Verification items for the finished model (mm, model axes). A direction names the side the tool comes from. Round coordinates to 2 decimals unless told otherwise and drop trailing zeros. Write each loop counter-clockwise with the first axis right and the second up, starting at its lowest first coordinate (ties: lowest second). Pieces come first, ordered by that corner, then holes. Notation, with made-up numbers: M -29,43 L 1,43 A10 cw 1,51 Z; hole C 89,86 d6. An arc over 180 degrees is marked long. Answer in a Markdown table with one row per item. Add a question column.
1. Sectioned sample at B-B on y = -3. Record the cut outline in (x, z).
2. Material ranges on probe 1 along X at (y, z) = (-22.5, 15); probe 2 along Y at (x, z) = (74, 22.5); probe 3 along X at (y, z) = (-13.5, 2), recorded low to high.
3. Sectioned sample at A-A on x = 75.5. Record the cut outline in (y, z).
4. Go/stop test with flat-tipped pins: pin 1 Ø10 at (x, y) = (48, -31.5) entering from +Z; pin 2 Ø10 at (x, y) = (40, -26) entering from +Z; pin 3 Ø19 at (x, y) = (54, -13) entering from -Z; pin 4 Ø6 at (y, z) = (-13, 31.5) entering from +X. Record where each tip stops, or that it passes through.
5. Sectioned sample at C-C on x = 17. Record the cut outline in (y, z), plus the area to 3 significant figures.
6. Sectioned sample at D-D on z = 24. Record the cut outline in (x, y) (3 decimals), plus the area to 3 significant figures.
7. Set-up check for faces 5 (the flat face through (67, -19, 25.718)), 6 (the flat face through (36, -38.1, 19)), 7 (the flat face through (66, -19, 13.018)): record each of +Z, -Z, +X, -X, +Y, -Y from which the full face is reachable in a straight line by a thin tool's end or side.
8. Draft check along Y on faces 1 (the cylindrical face through (76.714, -10.348, 19.279)), 2 (the cylindrical face through (18.611, -21.525, 18.783)), 3 (the flat face through (36, 0, 19)), 4 (the flat face through (38.1, -19, 32)). Enter one of: pulls with the +Y half, pulls with the -Y half, needs draft (parallel to the pull), parting line crosses it, or undercut.
```python
from build123d import *

# Parameters (mm, degrees)
F1_DEPTH = 38.1
F3_D     = 6.7564
F5_D     = 6.35


# Not quite as in the source:
# - the program builds the solid bodies; features that only make, move or delete a surface that nothing else refers to are left out


with BuildPart() as f1:
    # F0 (on Front) → F1 (new body)
    with BuildSketch(Plane.XZ):
        Polygon((0, 38.1), (0, 0), (38.1, 0), (38.1, 13.0175009682), (95.25, 13.0175009682), (95.25, 25.7175009682), (38.1, 25.7175009682), (38.1, 38.1), align=None)
    extrude(amount=F1_DEPTH)

    # F3 (through all)
    with Locations(Plane.XY.offset(38.1)):
        with Locations((17.8784132004, -18.2269066572)):
            Hole(F3_D / 2)

    # F5 (through all)
    with Locations(Plane.XY.offset(25.7175009682)):
        with Locations((54.4917780221, -10.4880234766), (54.4917780221, -23.1880234766), (73.5417780221, -23.1880234766), (73.5417780221, -10.4880234766)):
            Hole(F5_D / 2)


solid = f1.part
```
Geometry check:
| question | item | result |
|---|---|---|
| 1 | outline | M 0,0 L 38.1,0 L 38.1,13.02 L 95.25,13.02 L 95.25,25.72 L 38.1,25.72 L 38.1,38.1 L 0,38.1 Z |
| 2 | probe 1 | x = 0 to 51.39, 57.59 to 70.44, 76.64 to 95.25 |
| 2 | probe 2 | y = -38.1 to -26.33, -20.05 to -13.63, -7.35 to 0 |
| 2 | probe 3 | x = 0 to 38.1 |
| 3 | outline | M -38.1,13.02 L -25.69,13.02 L -25.69,25.72 L -38.1,25.72 Z; M -20.69,13.02 L -12.99,13.02 L -12.99,25.72 L -20.69,25.72 Z; M -7.99,13.02 L 0,13.02 L 0,25.72 L -7.99,25.72 Z |
| 4 | pin 1 | stops at z = 25.72 |
| 4 | pin 2 | stops at z = 38.1 |
| 4 | pin 3 | stops at z = 13.02 |
| 4 | pin 4 | stops at x = 38.1 |
| 5 | outline | M -38.1,0 L -21.49,0 L -21.49,38.1 L -38.1,38.1 Z; M -14.96,0 L 0,0 L 0,38.1 L -14.96,38.1 Z |
| 5 | area | 1,200 mm2 |
| 6 | outline | M 0,-38.1 L 95.25,-38.1 L 95.25,0 L 0,0 Z; hole C 17.878,-18.227 d6.756; hole C 54.492,-23.188 d6.35; hole C 54.492,-10.488 d6.35; hole C 73.542,-23.188 d6.35; hole C 73.542,-10.488 d6.35 |
| 6 | area | 3,470 mm2 |
| 7 | face 5 | +Z, +X, +Y, -Y |
| 7 | face 6 | +Z, -Z, +X, -X, -Y |
| 7 | face 7 | -Z, +X, +Y, -Y |
| 8 | face 1 | undercut |
| 8 | face 2 | undercut |
| 8 | face 3 | pulls with the +Y half |
| 8 | face 4 | needs draft |
